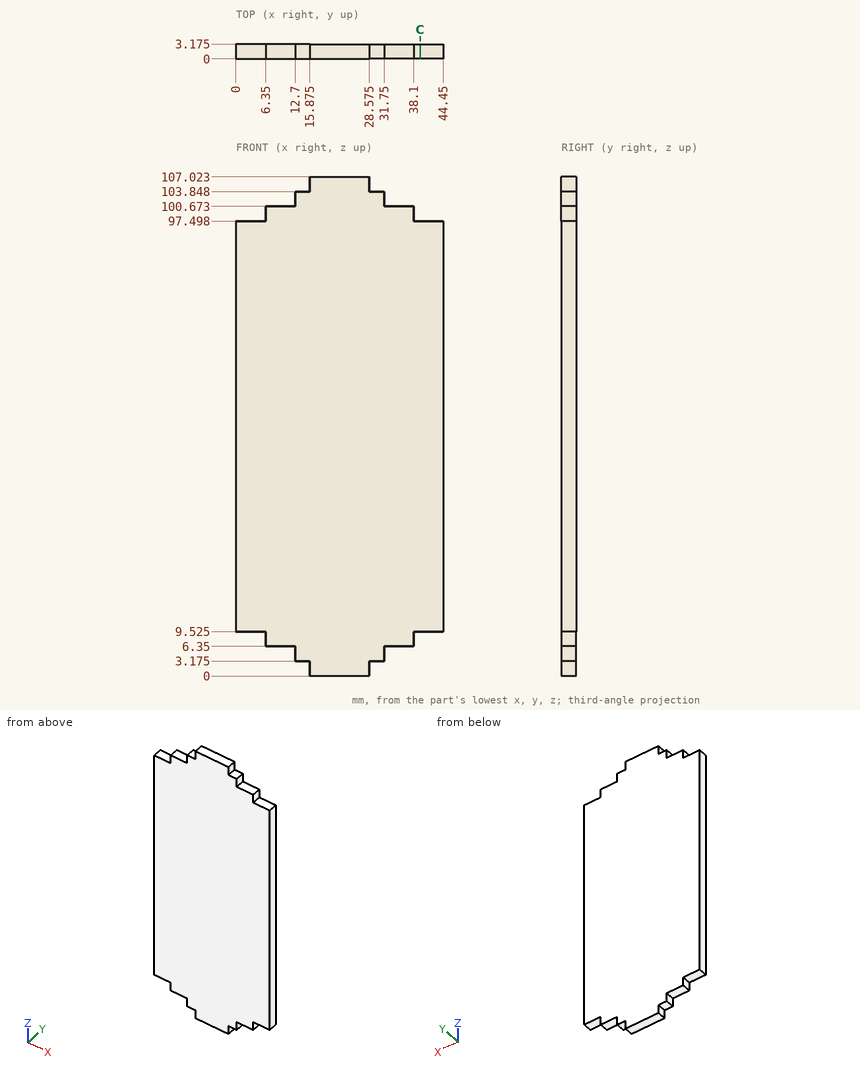
Answer from the drawing. Dimensions are ordinates in mm from the lowest x, y and z of the part. Give positions to 0.01 mm unless a question says otherwise; leave off trailing zeros. Loops run counter-clockwise (first coordinate to the right, second up) from the corner with the lowest first, then second, coordinate; pieces in that order, holes last. Notation, with made-up numbers: (-21, 31.25) -> (30, 31.25) arc R17 cw to (30, 43.25) -> close; hole circle Ø1 at (-26.5, 48). An arc over 180 degrees is marked (long way). Use a Markdown table: item, result.
Q1. Each of these flat-tipped pins is pushed along its axis until it touches: pin 1 (1.6 mm diameter, centred on y = 1.5, z = 99, fed in from -X); pin 2 (1 mm diameter, centred on x = 34.5, y = 1.5, fed in from +Z); pin 3 (1 mm diameter, centred on y = 1, z = 105, fed in from +X) (1 decimal). Where does it stop, or does it pass through?
Solved:
| item | result |
|---|---|
| pin 1 | stops at x = 6.35 |
| pin 2 | stops at z = 100.67 |
| pin 3 | stops at x = 28.6 |
Q2. Section C-C, the plane x = 39.5 is taken. Determine the outline of the cut face in (y, z) (1 decimal), then the cut area to 3 significant figures.
Solved:
| item | result |
|---|---|
| outline | (0, 9.5) -> (3.2, 9.5) -> (3.2, 97.5) -> (0, 97.5) -> close |
| area | 279 mm^2 |
Q3. Find the intervals of material crossed by line 1 along Z through (x, y) = (33, 0.35); line 2 along Z through (x, y) = (5, 0.8) (1 decimal), in increasing order.
Solved:
| item | result |
|---|---|
| line 1 | z = 6.35 to 100.67 |
| line 2 | z = 9.5 to 97.5 |
